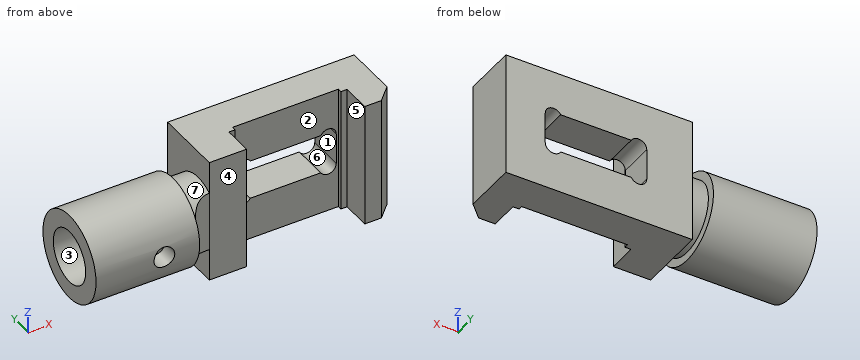
Autodesk Inventor part; units mm, degrees
ref_plane "Plan de construction1" through (90, 28, -30) normal (0, 0, 1) x (1, 0, 0)
ref_plane "Plan de construction2" through (18, -5, 0) normal (0, 0, 1) x (1, 0, 0)
ref_plane "Plan de construction3" through (-37, 4, 0) normal (0, -1, 0) x (1, 0, 0)
ref_plane "Plan de construction1" through (90, 28, -30) normal (0, 0, 1) x (1, 0, 0)
sketch "Esquisse1" plane through (90, 28, -30) normal (0, 0, 1) x (1, 0, 0)
  line L0 (0, 0) -> (-90, 0)
  line L1 (0, 0) -> (0, -26)
  line L2 (0, -26) -> (-7, -33)
  line L3 (-7, -33) -> (-15, -33)
  line L4 (-15, -19) -> (-15, -33)
  line L5 (-15, -19) -> (-18, -19)
  line L6 (-69, -17) -> (-18, -17)
  line L7 (-72, -19) -> (-69, -19)
  line L8 (-72, -33) -> (-72, -19)
  line L9 (-90, -33) -> (-72, -33)
  line L10 (-90, -33) -> (-90, 0)
  line L11 (-69, -17) -> (-69, -19)
  line L12 (-18, -17) -> (-18, -19)
  dimension "d10" = 17
  dimension "d11" = 16
  dimension "d12" = 18
  dimension "d13" = 15
  dimension "d14" = 3
  dimension "d15" = 2
  dimension "d17" = 3
  dimension "d18" = 2
  dimension "d19" = 51
extrude "Extrusion1" add sketch "Esquisse1" along normal blind 60
sketch "Esquisse2" plane through (21, 11, -30) normal (0, -1, 0) x (1, 0, 0)
  line L0 (42.535898, 20.5) -> (8.464102, 20.5)
  line L1 (8.464102, 39.5) -> (42.535898, 39.5)
  arc A0 (50, 37.5) -> (42.535898, 39.5) centre (46, 37.5) ccw
  arc A1 (42.535898, 20.5) -> (50, 22.5) centre (46, 22.5) ccw
  line L2 (50, 37.5) -> (50, 22.5)
  arc A2 (8.464102, 39.5) -> (1, 37.5) centre (5, 37.5) ccw
  line L3 (1, 22.5) -> (1, 37.5)
  arc A3 (1, 22.5) -> (8.464102, 20.5) centre (5, 22.5) ccw
  line L4 (51, 60) -> (0, 60)
  line L5 (0, 0) -> (0, 60)
  line L6 (0, 0) -> (51, 0)
  line L7 (51, 0) -> (51, 60)
extrude "Extrusion2" cut sketch "Esquisse2" against normal through all contours L0 A3 L3 A2 L1 A0 L2 A1
ref_plane "Plan de construction2" through (18, -5, 0) normal (0, 0, 1) x (1, 0, 0)
sketch "Esquisse3" plane through (18, -5, 0) normal (0, 0, 1) x (1, 0, 0)
  line L0 (-80, 34) -> (-80, -16)
  line L1 (-42, -7.5) -> (-42, 21.8)
  line L2 (-80, 9) -> (-42, 9)
  line L3 (-42, 9) -> (-42, 21.8)
  line L4 (-42, 21.8) -> (-80, 21.8)
  line L5 (-80, 21.8) -> (-80, 9)
  line L6 (-30, -12) -> (-30, 26)
  line L7 (-80, 9) -> (-30, 9)
  line L8 (-30, 9) -> (-30, -12)
  line L9 (-30, -12) -> (-80, -12)
  line L10 (-80, -12) -> (-80, 9)
  line L11 (-18, 0) -> (-18, 26)
  line L12 (-30, 9) -> (-18, 9)
  line L13 (-18, 9) -> (-18, 26)
  line L14 (-18, 26) -> (-30, 26)
  line L15 (-30, 26) -> (-30, 9)
  line L16 (0, 14) -> (0, 0)
  line L17 (0, 7) -> (-22.134302, 7)
  line L18 (-18, 0) -> (-18, 33)
  dimension "d20" = 21
  dimension "d21" = 12.8
  dimension "d22" = 12
  dimension "d23" = 62
  dimension "d24" = 17
  dimension "d29" = 2
  dimension "d30" = 38
revolve "Révolution1" add sketch "Esquisse3" angle 360 about axis through (-62, 4, 0) along (1, 0, 0) contours L6 L14 L11 L12 | L2 L7 L6 L9 L0
revolve "Révolution2" cut sketch "Esquisse3" angle 360 about axis through (-62, 4, 0) along (1, 0, 0) contours L4 L1 L2 L0
sketch "Esquisse5" plane through (18, -5, 0) normal (0, 0, 1) x (1, 0, 0)
  arc A0 (-18, 0) -> (-30, -12) centre (-18, -12) ccw
  line L0 (-18, 0) -> (-18, 0)
  line L1 (-30, 9) -> (-18, 9)
  line L2 (-18, -8) -> (-18, 0)
  line L3 (-18, -12) -> (-30, -12)
  line L4 (-18, 0) -> (0, 0)
  line L5 (-30, -8) -> (-30, 26)
  dimension "d31" = 12
sketch "Esquisse5 outline for Extrusion3" plane through (18, -5, 0) normal (0, 0, 1) x (1, 0, 0)
  arc A0 (-18, 0) -> (-30, -12) centre (-18, -12) ccw
  line L0 (-18, -8) -> (-18, 0)
  line L1 (-30, -12) -> (-18, -8)
extrude "Extrusion3" cut sketch "Esquisse5 outline for Extrusion3" along normal through all both and the other way through all
ref_plane "Plan de construction3" through (-37, 4, 0) normal (0, -1, 0) x (1, 0, 0)
sketch "Esquisse6" plane through (-37, 4, 0) normal (0, -1, 0) x (1, 0, 0)
  arc A0 (5.953227, 4.562013) -> (11.578201, 3.492329) centre (7.999875, -0.000026) ccw
  circle A1 centre (7.999875, -0.000026) radius 5.000096
  dimension "d26" = 5.0001
extrude "Extrusion4" cut sketch "Esquisse6" along normal through all
sketch "Esquisse7" plane through (-24, 4, 0) normal (-1, 0, 0) x (0, 0, 1)
  circle A0 centre (0, 0) radius 12.8
hole "Perçage1" at (-24, 4, 0) direction (1, 0, 0) diameter 4.134 depth 19.5 tip angle 118 counterbore diameter 8 counterbore depth 4.5
sketch "Esquisse8" plane through (-24, 4, 0) normal (-1, 0, 0) x (0, 0, 1)
  circle A0 centre (0, 0) radius 4
  circle A1 centre (0, 0) radius 12.8
  line L0 (-12.8, 0) -> (12.8, 0)
properties part number "crosse" material "Acier doux"
Work out the finished part from the listing and answer in its coordinate system (mm). Face numbers are marked on the shaded views. A direction names the side the tool comes from. Give positions to 0.01 mm unless a question says otherwise; leave off trailing zeros. Order: outer loops, then holes, each group sorted by start corner. A loop starts at its lowest first (then second) coordinate and runs counter-clockwise, first axis right, second up.
1. Section D-D, the plane x = 7.5 is taken. Determine the outline of the cut face in (y, z), and give its area (3 significant figures).
Result sheet:
outline: (-5, -30) - (28, -30) - (28, 30) - (-5, 30) - close
area: 1,980 mm2
2. Section A-A, the plane x = 62 is taken. Determine the outline of the cut face in (y, z).
Result sheet:
outline: (11, -30) - (28, -30) - (28, -9.5) - (11, -9.5) - close; (11, 9.5) - (28, 9.5) - (28, 30) - (11, 30) - close
3. Each of these flat-tipped pins is pushed along its axis until it touches: P1, Ø5, axis at x = -20.5, y = 1, coming from the -Z side; P2, Ø9, axis at x = 79, z = -2, coming from the -Y side; P3, Ø3.5, axis at y = 4, z = 0, coming from the -X side; P4, Ø6, axis at y = -6.5, z = -4.5, coming from the -X side. Where does it stop, or does it pass through?
Result sheet:
P1: stops at z = -20.99
P2: stops at y = -5
P3: stops at x = -4.31
P4: stops at x = -62
4. Section C-C, the plane x = -38 is taken. Determine the outline of the cut face in (y, z).
Result sheet:
outline: circle Ø42 at (4, 0); hole circle Ø25.6 at (4, 0)
5. For the marked faces 4, 5, 6 and 7, determine the directions among +Z, -Z, +X, -X, +Y, -Y from which every point of the face is accessible in a straight line to the end or side of a thin tool.
Result sheet:
face 4: +Z, -Z, +X, -Y
face 5: +Z, -Z, -Y
face 6: +Y, -Y
face 7: none
6. The mould has two halves that part along Y. Classify the marked faces 1, 2 and 3: released by +Y, released by -Y, zero draft, split by the parting line, or undercut.
Result sheet:
face 1: zero draft
face 2: released by -Y
face 3: undercut
7. Straight lines are drawn through the part: L1, parallel to X at y = 20, z = -7; L2, parallel to X at y = 4.5, z = 19; L3, parallel to X at y = 3.5, z = -5. For each, find the intervals that lie inside material, in ascending order.
Result sheet:
L1: x = -62 to -12, 0 to 22, 71 to 90
L2: x = -62 to -12, 0 to 18, 75 to 90
L3: x = -24 to 18, 75 to 90
8. Section B-B, the plane y = 23.5 is taken. Determine the outline of the cut face in (x, z), and give its area (3 significant figures).
Result sheet:
outline: (-62, -7.79) - (-12, -7.79) - (-12, 7.79) - (-62, 7.79) - close; (0, -30) - (90, -30) - (90, 30) - (0, 30) - close; hole (22, -7.5) arc R4 ccw to (29.46, -9.5) - (63.54, -9.5) arc R4 ccw to (71, -7.5) - (71, 7.5) arc R4 ccw to (63.54, 9.5) - (29.46, 9.5) arc R4 ccw to (22, 7.5) - close
area: 5,210 mm2
